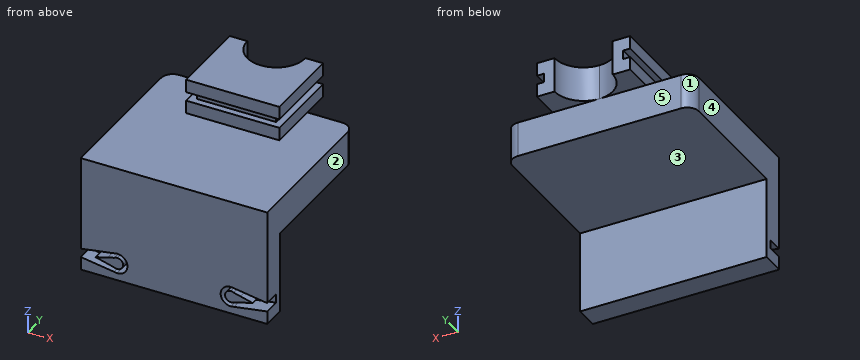
```python
from build123d import *

# Parameters (mm, degrees)
BOSS_EXTRUDE4_DEPTH = 19.05
SKETCH4_W           = 101.6
SKETCH4_H           = 19.05
BOSS_EXTRUDE7_DEPTH = 12.7
SKETCH5_W           = 101.6
SKETCH5_H           = 12.7
BOSS_EXTRUDE8_DEPTH = 44.45
CUT_EXTRUDE1_DEPTH  = 8.89
BOSS_EXTRUDE9_DEPTH = 19.05
SKETCH9_W           = 4.826
SKETCH9_H           = 44.053125
CUT_EXTRUDE2_DEPTH  = 3.81
SKETCH10_W          = 46.99
SKETCH10_H          = 4.826
CUT_EXTRUDE3_DEPTH  = 3.81
SKETCH11_W          = 4.826
SKETCH11_H          = 40.243125
CUT_EXTRUDE4_DEPTH  = 3.81


with BuildPart() as part:
    # Sketch1 → Boss-Extrude4 (new body)
    with BuildSketch(Plane.XY):
        with BuildLine():
            Line((-109.851890308, -12.598485557), (-109.851890308, -18.948485557))
            Line((-109.851890308, -18.948485557), (-103.501890308, -18.948485557))
            Line((-103.501890308, -18.948485557), (-14.601890308, -18.948485557))
            Line((-14.601890308, -18.948485557), (-8.251890308, -18.948485557))
            Line((-8.251890308, -18.948485557), (-8.251890308, -12.598485557))
            Line((-8.251890308, -12.598485557), (-8.251890308, 49.314014443))
            ThreePointArc((-8.251890308, 49.314014443), (-10.111762247, 53.804142503), (-14.601890308, 55.664014443))
            Line((-14.601890308, 55.664014443), (-103.501890308, 55.664014443))
            ThreePointArc((-103.501890308, 55.664014443), (-107.992018368, 53.804142503), (-109.851890308, 49.314014443))
            Line((-109.851890308, 49.314014443), (-109.851890308, -12.598485557))
        make_face()
    extrude(amount=BOSS_EXTRUDE4_DEPTH)

    # Sketch4 → Boss-Extrude7 (add)
    with BuildSketch(Plane(origin=(0, -18.948485557, 0), x_dir=(-1, 0, 0), z_dir=(0, -1, 0))):
        with Locations((59.051890308, -9.525)):
            Rectangle(SKETCH4_W, SKETCH4_H)
    extrude(amount=BOSS_EXTRUDE7_DEPTH)

    # Sketch5 → Boss-Extrude8 (add)
    with BuildSketch(Plane(origin=(0, 0, 0), x_dir=(-1, 0, 0), z_dir=(0, 0, -1))):
        with Locations((59.051890308, -25.298485557)):
            Rectangle(SKETCH5_W, SKETCH5_H)
    extrude(amount=BOSS_EXTRUDE8_DEPTH)

    # Sketch7 → Cut-Extrude1 (cut)
    with BuildSketch(Plane.XZ.offset(31.648485557)):
        with BuildLine():
            Line((-26.362020963, -40.203870905), (-8.251890308, -37.30625))
            Line((-8.251890308, -37.30625), (-8.251890308, -32.54375))
            Line((-8.251890308, -32.54375), (-26.362020963, -29.646129095))
            ThreePointArc((-26.362020963, -29.646129095), (-24.177794705, -30.985152301), (-22.826560616, -33.161845648))
            Line((-22.826560616, -33.161845648), (-16.246378994, -34.925))
            Line((-16.246378994, -34.925), (-22.826560616, -36.688154352))
            ThreePointArc((-22.826560616, -36.688154352), (-24.177794705, -38.864847699), (-26.362020963, -40.203870905))
        make_face()
        with BuildLine():
            Line((-28.095640308, -40.48125), (-26.362020963, -40.203870905))
            ThreePointArc((-26.362020963, -40.203870905), (-24.177794705, -38.864847699), (-22.826560616, -36.688154352))
            Line((-22.826560616, -36.688154352), (-26.508140308, -37.674630657))
            ThreePointArc((-26.508140308, -37.674630657), (-27.27388984, -37.991814498), (-28.095640308, -38.1))
            ThreePointArc((-28.095640308, -38.1), (-31.270640308, -34.925), (-28.095640308, -31.75))
            ThreePointArc((-28.095640308, -31.75), (-27.27388984, -31.858185502), (-26.508140308, -32.175369343))
            Line((-26.508140308, -32.175369343), (-22.826560616, -33.161845648))
            ThreePointArc((-22.826560616, -33.161845648), (-24.177794705, -30.985152301), (-26.362020963, -29.646129095))
            Line((-26.362020963, -29.646129095), (-28.095640308, -29.36875))
            ThreePointArc((-28.095640308, -29.36875), (-33.651890308, -34.925), (-28.095640308, -40.48125))
        make_face()
        with BuildLine():
            Line((-109.851890308, -32.54375), (-109.851890308, -37.30625))
            Line((-109.851890308, -37.30625), (-91.741759653, -40.203870905))
            ThreePointArc((-91.741759653, -40.203870905), (-93.925985911, -38.864847699), (-95.277219999, -36.688154352))
            Line((-95.277219999, -36.688154352), (-101.857401622, -34.925))
            Line((-101.857401622, -34.925), (-95.277219999, -33.161845648))
            ThreePointArc((-95.277219999, -33.161845648), (-93.925985911, -30.985152301), (-91.741759653, -29.646129095))
            Line((-91.741759653, -29.646129095), (-109.851890308, -32.54375))
        make_face()
        with BuildLine():
            ThreePointArc((-95.277219999, -36.688154352), (-93.925985911, -38.864847699), (-91.741759653, -40.203870905))
            Line((-91.741759653, -40.203870905), (-90.008140308, -40.48125))
            ThreePointArc((-90.008140308, -40.48125), (-86.079278255, -38.853862053), (-84.451890308, -34.925))
            ThreePointArc((-84.451890308, -34.925), (-86.079278255, -30.996137947), (-90.008140308, -29.36875))
            Line((-90.008140308, -29.36875), (-91.741759653, -29.646129095))
            ThreePointArc((-91.741759653, -29.646129095), (-93.925985911, -30.985152301), (-95.277219999, -33.161845648))
            Line((-95.277219999, -33.161845648), (-91.595640308, -32.175369343))
            ThreePointArc((-91.595640308, -32.175369343), (-90.829890776, -31.858185502), (-90.008140308, -31.75))
            ThreePointArc((-90.008140308, -31.75), (-87.763076278, -32.67993597), (-86.833140308, -34.925))
            ThreePointArc((-86.833140308, -34.925), (-87.763076278, -37.17006403), (-90.008140308, -38.1))
            ThreePointArc((-90.008140308, -38.1), (-90.829890776, -37.991814498), (-91.595640308, -37.674630657))
            Line((-91.595640308, -37.674630657), (-95.277219999, -36.688154352))
        make_face()
    extrude(amount=-CUT_EXTRUDE1_DEPTH, mode=Mode.SUBTRACT)

    # Sketch3 → Boss-Extrude9 (add)
    with BuildSketch(Plane.XY.offset(19.05)):
        with BuildLine():
            Line((-84.451890308, 71.539014443), (-84.451890308, 55.664014443))
            Line((-84.451890308, 55.664014443), (-59.05189022, 55.664014443))
            ThreePointArc((-59.05189022, 55.664014443), (-70.277210428, 60.31369426), (-74.926890308, 71.539014443))
            Line((-74.926890308, 71.539014443), (-84.451890308, 71.539014443))
        make_face()
        Polygon((-84.451890308, 55.664014443), (-84.451890308, 27.485889443), (-33.651890308, 27.485889443), (-33.651890308, 55.664014443), (-59.05189022, 55.664014443), align=None)
        with BuildLine():
            Line((-59.05189022, 55.664014443), (-33.651890308, 55.664014443))
            Line((-33.651890308, 55.664014443), (-33.651890308, 71.539014443))
            Line((-33.651890308, 71.539014443), (-43.176890308, 71.539014443))
            ThreePointArc((-43.176890308, 71.539014443), (-47.826570125, 60.313694322), (-59.05189022, 55.664014443))
        make_face()
    extrude(amount=BOSS_EXTRUDE9_DEPTH)

    # Sketch9 → Cut-Extrude2 (cut)
    with BuildSketch(Plane(origin=(-33.651890308, 0, 0), x_dir=(0, 0, -1), z_dir=(1, 0, 0))):
        with Locations((-28.575, 49.512451943)):
            Rectangle(SKETCH9_W, SKETCH9_H)
    extrude(amount=-CUT_EXTRUDE2_DEPTH, mode=Mode.SUBTRACT)

    # Sketch10 → Cut-Extrude3 (cut)
    with BuildSketch(Plane.XZ.offset(-27.485889443)):
        with Locations((-60.956890308, 28.575)):
            Rectangle(SKETCH10_W, SKETCH10_H)
    extrude(amount=-CUT_EXTRUDE3_DEPTH, mode=Mode.SUBTRACT)

    # Sketch11 → Cut-Extrude4 (cut)
    with BuildSketch(Plane.ZY.offset(84.451890308)):
        with Locations((28.575, 51.417451943)):
            Rectangle(SKETCH11_W, SKETCH11_H)
    extrude(amount=-CUT_EXTRUDE4_DEPTH, mode=Mode.SUBTRACT)


solid = part.part
```
Geometry check sheet. Reference: the model listing, model coordinates, mm. Face numbers are marked on the shaded views. A direction names the side the tool comes from. Coordinates: 2 decimals unless noted, no trailing zeros. Write each loop counter-clockwise with the first axis right and the second up, starting at its lowest first coordinate (ties: lowest second). Pieces come first, ordered by that corner, then holes. Notation, with made-up numbers: M -1.75,0 L 47.25,0 A21 cw 47.25,7 Z; hole C -28.75,56 d8. An arc over 180 degrees is marked long. Use one line per item in the form item = value. Start each with the question number.
1) Section check C-C on y = 45. Enter the section's corners in (x, z).
2) Set-up check for the marked faces 4 and 5: record each of +Z, -Z, +X, -X, +Y, -Y from which the full face is reachable in a straight line by a thin tool's end or side.
3) Release check for a two-part mould opening along X. For the marked faces 1, 2 and 3 record: pulls with the +X half, pulls with the -X half, needs draft (parallel to the pull), parting line crosses it, or undercut.
4) Thickness scan on probe 1 along Z at (x, y) = (-32, 47); probe 2 along Z at (x, y) = (-66.5, 35.5); probe 3 along Y at (x, z) = (-54.5, -5). Record the ranges inside material, lowest first. Write a range as from..to.
5) Section check D-D on z = 23. Enter the section's corners in (x, y) (3 decimals), and give its area (3 significant figures).
6) Section check A-A on x = -83. Enter the section's corners in (y, z), and give its area (3 significant figures).
7) Go/stop test with flat-tipped pins: pin 1 Ø12 at (x, y) = (-57, -15) entering from -Z; pin 2 Ø3 at (x, z) = (-23, -13) entering from +Y; pin 3 Ø5.5 at (y, z) = (45, 23.5) entering from +X; pin 4 Ø4 at (y, z) = (46, 28) entering from -X. Record where each tip stops, or that it passes through.
8) Section check B-B on y = 57. Enter the section's corners in (x, z).
Responses:
q1.outline = M -109.85,0 L -8.25,0 L -8.25,19.05 L -33.65,19.05 L -33.65,26.16 L -37.46,26.16 L -37.46,30.99 L -33.65,30.99 L -33.65,38.1 L -84.45,38.1 L -84.45,30.99 L -80.64,30.99 L -80.64,26.16 L -84.45,26.16 L -84.45,19.05 L -109.85,19.05 Z
q2.face_4 = +Z, -Z, -X, +Y, -Y
q2.face_5 = -Z, +X, -X, +Y
q3.face_1 = pulls with the -X half
q3.face_2 = pulls with the +X half
q3.face_3 = needs draft
q4.probe_1 = 0..19.05
q4.probe_2 = 0..38.1
q4.probe_3 = -31.65..-18.95
q5.outline = M -84.452,27.486 L -33.652,27.486 L -33.652,71.539 L -43.177,71.539 A15.875 cw -74.927,71.539 L -84.452,71.539 Z
q5.area = 1,840 mm2
q6.outline = M -31.65,-44.45 L -18.95,-44.45 L -18.95,0 L 55.66,0 L 55.66,19.05 L 71.54,19.05 L 71.54,26.16 L 27.49,26.16 L 27.49,19.05 L -31.65,19.05 Z; M 27.49,30.99 L 71.54,30.99 L 71.54,38.1 L 27.49,38.1 Z
q6.area = 2,850 mm2
q7.pin_1 = -44.45
q7.pin_2 = -18.95
q7.pin_3 = -33.65
q7.pin_4 = -84.45
q8.outline = M -84.45,19.05 L -65.43,19.05 L -65.43,38.1 L -84.45,38.1 L -84.45,30.99 L -80.64,30.99 L -80.64,26.16 L -84.45,26.16 Z; M -52.68,19.05 L -33.65,19.05 L -33.65,26.16 L -37.46,26.16 L -37.46,30.99 L -33.65,30.99 L -33.65,38.1 L -52.68,38.1 Z
